Work out the finished part from the listing and answer in its coordinate system (mm). A direction names the side the tool comes from. Coordinates: 2 decimals unless noted, no trailing zeros. Order: outer loops, then holes, each group sorted by start corner. A loop starts at its lowest first (then second) coordinate and runs counter-clockwise, first axis right, second up. Notation, with made-up numbers: M 76,-35.5 L 113,-35.5 A21 ccw 113,-4.5 Z; hole C 65.5,89.5 d11. An arc over 180 degrees is marked long. Use a Markdown table: item, result. Add a question column.
from build123d import *

# Parameters (mm, degrees)
F0_W     = 127
F0_H     = 76.2
F1_DEPTH = 30
F2_R     = 5
F3_W     = 7
F3_H     = 13.8
F4_DEPTH = 16.4
F5_W     = 7
F5_H     = 13.8
F6_DEPTH = 16.4


with BuildPart() as f1:
    # F0 (on Front) → F1 (new body)
    with BuildSketch(Plane.XZ):
        Rectangle(F0_W, F0_H)
    extrude(amount=F1_DEPTH)

    # F2
    f2_edges = [f1.edges().sort_by_distance(p)[0] for p in [
        (0, -30, 38.1),
        (0, 0, 38.1),
        (0, -30, -38.1),
        (0, 0, -38.1),
    ]]
    fillet(f2_edges, radius=F2_R)

    # F3 (on face) → F4 (cut)
    with BuildSketch(Plane.YZ.offset(63.5)):
        with Locations((-14.062501, 18.641072)):
            Rectangle(F3_W, F3_H)
    extrude(amount=-F4_DEPTH, mode=Mode.SUBTRACT)

    # F5 (on face) → F6 (cut)
    with BuildSketch(Plane.YZ.offset(63.5)):
        with Locations((-14.062501, 0.937244)):
            Rectangle(F5_W, F5_H)
    extrude(amount=-F6_DEPTH, mode=Mode.SUBTRACT)


solid = f1.part
(1) A cutting plane is placed at B-B on y = -2. Write down the section's boundary in (x, z).
(2) Which of the six approach directions +Z, -Z, +X, -X, +Y, -Y give full straight-line access (tool end or side, diameter ignored) to faces 5 (the flat face through (55, -14, -5.963)), 6 (the flat face through (63.5, -18, -1))?
(3) A cutting plane is placed at A-A on z = 1.5. Write down the section's boundary in (x, y), plus the area to 3 significant figures.
(4) The mould has two halves that part along Z. Classify faces 1 (the cylindrical face through (0.89, -1.5, -36.67)), 2 (the flat face through (47.1, -14, 1)), 3 (the flat face through (-1, 0, 0)), 4 (the flat face through (55, -10.563, 19)): pulls with the +Z half, pulls with the -Z half, needs draft (parallel to the pull), parting line crosses it, or undercut.
(5) Given P1, Ø3.5, axis at y = -14.5, z = 18.5, coming from the +X side, flat-ended and moving along its own axis, determine where the tip first touches the part or whether it passes through.
(6) Straight lines are drawn through the part: line 1 (Y direction, x = 54, z = 1); line 2 (Z direction, x = 51.5, y = -12.25); line 3 (X direction, y = -15.5, z = 19.5). For each, find the intervals that lie inside material, in ascending order.
From the geometry:
| question | item | result |
|---|---|---|
| 1 | outline | M -63.5,-37.1 L 63.5,-37.1 L 63.5,37.1 L -63.5,37.1 Z |
| 2 | face 5 | +X |
| 2 | face 6 | +Z, -Z, +X, +Y, -Y |
| 3 | outline | M -63.5,-30 L 63.5,-30 L 63.5,-17.56 L 47.1,-17.56 L 47.1,-10.56 L 63.5,-10.56 L 63.5,0 L -63.5,0 Z |
| 3 | area | 3,700 mm2 |
| 4 | face 1 | pulls with the -Z half |
| 4 | face 2 | undercut |
| 4 | face 3 | needs draft |
| 4 | face 4 | undercut |
| 5 | P1 | stops at x = 47.1 |
| 6 | line 1 | y = -30 to -17.56, -10.56 to 0 |
| 6 | line 2 | z = -38.1 to -5.96, 7.84 to 11.74, 25.54 to 38.1 |
| 6 | line 3 | x = -63.5 to 47.1 |
